Input: part model. Units: mm. Frame: model coordinates. Face numbers are marked on the shaded views. A direction names the side the tool comes from. Round coordinates to 2 decimals unless told otherwise and drop trailing zeros. Order: outer loops, then holes, each group sorted by start corner. A loop starts at its lowest first (then second) coordinate and runs counter-clockwise, first axis right, second up.
Item 1: Cut plane D-D on z = 14. Output: boundary loops of the cut face in (x, y), then the cut area to 3 significant figures.
Item 2: Cut plane B-B on x = 55. Output: boundary loops of the cut face in (y, z).
Item 3: Cut plane C-C on x = -35. Output: boundary loops of the cut face in (y, z).
Item 4: Cut plane A-A on y = -8. Output: boundary loops of the cut face in (x, z).
Item 5: Line query: L1, parallel to X at y = -1.35, z = 44.5; L2, parallel to X at y = -2.05, z = -48.5; L3, parallel to X at y = -8, z = -63.25. Output: solid intervals per line, ascending.
Item 6: Reachability of the marked faces 1 and 2 from +Z, -Z, +X, -X, +Y, -Y: full face, straight path, thin tool, end or side. Return the list, or none.
Item 7: First-contact query: pin 1 (4.5 mm diameter, centred on x = -55, y = 5, fed in from -Z); pin 2 (10 mm diameter, centred on x = 65.5, z = -48.5, fed in from -Y); pin 3 (2.5 mm diameter, centred on x = -5, y = -1.5, fed in from +Z); pin 4 (3 mm diameter, centred on x = -76, z = 44.5, fed in from +Y). Flat tips, straight axial feed; report the tip coordinate or a pass-through.
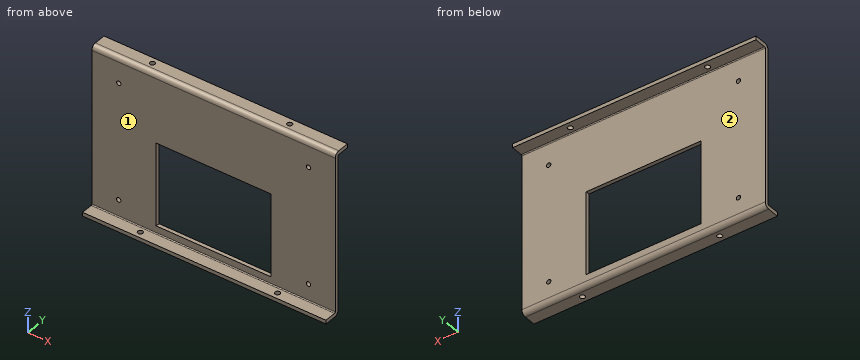
```python
from build123d import *

# Parameters (mm, degrees)
SKETCH_1_W                       = 195
SKETCH_1_H                       = 130
SM_BASE_FLANGE_1_DEPTH           = 3
SM_EDGE_FLANGE_1_STRIP_W         = 13.4732
SM_EDGE_FLANGE_1_STRIP_H         = 3
SM_EDGE_FLANGE_1_STRIP_CUT_DEPTH = 195
SM_EDGE_FLANGE_1_DEPTH           = 195
SM_EDGE_FLANGE_2_STRIP_W         = 13.4732
SM_EDGE_FLANGE_2_STRIP_H         = 3
SM_EDGE_FLANGE_2_STRIP_CUT_DEPTH = 195
SM_EDGE_FLANGE_2_DEPTH           = 195
SKETCH_12_R                      = 2
CUT_EXTRUDE_1_DEPTH              = 10
SKETCH_13_R                      = 2
CUT_EXTRUDE_2_DEPTH              = 10
CUT_EXTRUDE_3_REACH              = 119.899
SKETCH_14_R                      = 1.75
SKETCH_14_W                      = 92
SKETCH_14_H                      = 66


# Sheet-metal steps are written as plain solids
with BuildPart() as part:
    # Sketch 1 → 基体-法兰1 (new body)
    with BuildSketch(Plane(origin=(0, 0, 0), x_dir=(1, 0, 0), z_dir=(0, 1, 0))):
        Rectangle(SKETCH_1_W, SKETCH_1_H)
    extrude(amount=-SM_BASE_FLANGE_1_DEPTH)

    # 边线-法兰1 strip (across the edge) → 边线-法兰1 strip cut (cut)
    with BuildSketch(Plane(origin=(-97.5, 0, 65), x_dir=(0, 0, -1), z_dir=(1, 0, 0))):
        with Locations((-3, -1.5)):
            Rectangle(SM_EDGE_FLANGE_1_STRIP_W, SM_EDGE_FLANGE_1_STRIP_H)
    extrude(amount=SM_EDGE_FLANGE_1_STRIP_CUT_DEPTH, mode=Mode.SUBTRACT)

    # 边线-法兰1 section (across the edge) → 边线-法兰1 (add)
    with BuildSketch(Plane(origin=(-97.5, 0, 65), x_dir=(0, 0, -1), z_dir=(1, 0, 0))):
        with BuildLine():
            Line((0, 0.7366), (0, 10))
            Line((0, 10), (3, 10))
            Line((3, 10), (3, 0.7366))
            ThreePointArc((3, 0.7366), (3.215745145, 0.215745145), (3.7366, 0))
            Line((3.7366, 0), (3.7366, -3))
            ThreePointArc((3.7366, -3), (1.094424801, -1.905575199), (0, 0.7366))
        make_face()
    extrude(amount=SM_EDGE_FLANGE_1_DEPTH)

    # 边线-法兰2 strip (across the edge) → 边线-法兰2 strip cut (cut)
    with BuildSketch(Plane(origin=(-97.5, -3, -65), x_dir=(0, 0, 1), z_dir=(1, 0, 0))):
        with Locations((-3, -1.5)):
            Rectangle(SM_EDGE_FLANGE_2_STRIP_W, SM_EDGE_FLANGE_2_STRIP_H)
    extrude(amount=SM_EDGE_FLANGE_2_STRIP_CUT_DEPTH, mode=Mode.SUBTRACT)

    # 边线-法兰2 section (across the edge) → 边线-法兰2 (add)
    with BuildSketch(Plane(origin=(-97.5, -3, -65), x_dir=(0, 0, 1), z_dir=(1, 0, 0))):
        with BuildLine():
            Line((0, 0.7366), (0, 10))
            Line((0, 10), (3, 10))
            Line((3, 10), (3, 0.7366))
            ThreePointArc((3, 0.7366), (3.215745145, 0.215745145), (3.7366, 0))
            Line((3.7366, 0), (3.7366, -3))
            ThreePointArc((3.7366, -3), (1.094424801, -1.905575199), (0, 0.7366))
        make_face()
    extrude(amount=SM_EDGE_FLANGE_2_DEPTH)

    # 草图12 → 切除-拉伸1 (cut)
    with BuildSketch(Plane.XY.offset(65)):
        with Locations((-55, 5)):
            Circle(SKETCH_12_R)
        with Locations(Location((55, 5, 0), (0, 0, 180))):
            Circle(SKETCH_12_R)
    extrude(amount=-CUT_EXTRUDE_1_DEPTH, mode=Mode.SUBTRACT)

    # 草图13 → 切除-拉伸2 (cut)
    with BuildSketch(Plane(origin=(0, 0, -65), x_dir=(-1, 0, 0), z_dir=(0, 0, -1))):
        with Locations(Location((-55, -8, 0), (0, 0, 90))):
            Circle(SKETCH_13_R)
        with Locations(Location((55, -8, 0), (0, 0, 270))):
            Circle(SKETCH_13_R)
    extrude(amount=-CUT_EXTRUDE_2_DEPTH, mode=Mode.SUBTRACT)

    # 草图14 → 切除-拉伸3 (cut, up to next)
    with BuildSketch(Plane(origin=(0, 0, 0), x_dir=(1, 0, 0), z_dir=(0, 1, 0)), mode=Mode.PRIVATE) as cut_extrude_3_sk1:
        with Locations(Location((-76, 48.5, 0), (0, 0, 270))):
            Circle(SKETCH_14_R)
    cut_extrude_3_tool1 = extrude(cut_extrude_3_sk1.sketch, amount=-CUT_EXTRUDE_3_REACH, mode=Mode.PRIVATE) & part.part
    # 草图14 → 切除-拉伸3 (cut, up to next)
    with BuildSketch(Plane(origin=(0, 0, 0), x_dir=(1, 0, 0), z_dir=(0, 1, 0)), mode=Mode.PRIVATE) as cut_extrude_3_sk2:
        with Locations(Location((76, 48.5, 0), (0, 0, 90))):
            Circle(SKETCH_14_R)
    cut_extrude_3_tool2 = extrude(cut_extrude_3_sk2.sketch, amount=-CUT_EXTRUDE_3_REACH, mode=Mode.PRIVATE) & part.part
    # 草图14 → 切除-拉伸3 (cut, up to next)
    with BuildSketch(Plane(origin=(0, 0, 0), x_dir=(1, 0, 0), z_dir=(0, 1, 0)), mode=Mode.PRIVATE) as cut_extrude_3_sk3:
        with Locations(Location((76, -44.5, 0), (0, 0, 270))):
            Circle(SKETCH_14_R)
    cut_extrude_3_tool3 = extrude(cut_extrude_3_sk3.sketch, amount=-CUT_EXTRUDE_3_REACH, mode=Mode.PRIVATE) & part.part
    # 草图14 → 切除-拉伸3 (cut, up to next)
    with BuildSketch(Plane(origin=(0, 0, 0), x_dir=(1, 0, 0), z_dir=(0, 1, 0)), mode=Mode.PRIVATE) as cut_extrude_3_sk4:
        with Locations(Location((-76, -44.5, 0), (0, 0, 90))):
            Circle(SKETCH_14_R)
    cut_extrude_3_tool4 = extrude(cut_extrude_3_sk4.sketch, amount=-CUT_EXTRUDE_3_REACH, mode=Mode.PRIVATE) & part.part
    # 草图14 → 切除-拉伸3 (cut, up to next)
    with BuildSketch(Plane(origin=(0, 0, 0), x_dir=(1, 0, 0), z_dir=(0, 1, 0)), mode=Mode.PRIVATE) as cut_extrude_3_sk5:
        with Locations((0, 23)):
            Rectangle(SKETCH_14_W, SKETCH_14_H)
    cut_extrude_3_tool5 = extrude(cut_extrude_3_sk5.sketch, amount=-CUT_EXTRUDE_3_REACH, mode=Mode.PRIVATE) & part.part
    add(cut_extrude_3_tool1.solids().sort_by_distance((-76, 0, -48.5))[0], mode=Mode.SUBTRACT)
    add(cut_extrude_3_tool2.solids().sort_by_distance((76, 0, -48.5))[0], mode=Mode.SUBTRACT)
    add(cut_extrude_3_tool3.solids().sort_by_distance((76, 0, 44.5))[0], mode=Mode.SUBTRACT)
    add(cut_extrude_3_tool4.solids().sort_by_distance((-76, 0, 44.5))[0], mode=Mode.SUBTRACT)
    add(cut_extrude_3_tool5.solids().sort_by_distance((0, 0, -23))[0], mode=Mode.SUBTRACT)


solid = part.part
```
From the geometry:
1. outline: (-97.5, -3) - (97.5, -3) - (97.5, 0) - (-97.5, 0) - close
1. area: 585 mm2
2. outline: (-13, -65) - (-10, -65) - (-10, -62) - (-13, -62) - close; (-6, -65) - (-3.74, -65) arc R3.74 ccw to (0, -61.26) - (0, 61.26) arc R0.74 cw to (0.74, 62) - (3, 62) - (3, 65) - (0.74, 65) arc R3.74 ccw to (-3, 61.26) - (-3, -61.26) arc R0.74 cw to (-3.74, -62) - (-6, -62) - close; (7, 62) - (10, 62) - (10, 65) - (7, 65) - close
3. outline: (-13, -65) - (-3.74, -65) arc R3.74 ccw to (0, -61.26) - (0, -56) - (-3, -56) - (-3, -61.26) arc R0.74 cw to (-3.74, -62) - (-13, -62) - close; (-3, 10) - (0, 10) - (0, 61.26) arc R0.74 cw to (0.74, 62) - (10, 62) - (10, 65) - (0.74, 65) arc R3.74 ccw to (-3, 61.26) - close
4. outline: (-97.5, -65) - (-57, -65) - (-57, -62) - (-97.5, -62) - close; (-53, -65) - (53, -65) - (53, -62) - (-53, -62) - close; (57, -65) - (97.5, -65) - (97.5, -62) - (57, -62) - close
5. L1: x = -97.5 to -77.75, -74.25 to 74.25, 77.75 to 97.5
5. L2: x = -97.5 to -77.75, -74.25 to -46, 46 to 74.25, 77.75 to 97.5
5. L3: x = -97.5 to -57, -53 to 53, 57 to 97.5
6. face 1: +Z, +X, -X, -Y
6. face 2: -Z, +X, -X, +Y
7. pin 1: stops at z = 62
7. pin 2: stops at y = -3
7. pin 3: stops at z = 64.87
7. pin 4: passes through
